from build123d import *

# Parameters (mm, degrees)
ESTRUSIONE_SOTTILE1_DEPTH    = 10
TAGLIO_ESTRUSIONE2_DEPTH     = 10
SCHIZZO3_R                   = 12.75
SCHIZZO3_R_2                 = 3.161562041
ESTRUSIONE_ESTRUSIONE1_DEPTH = 10


with BuildPart() as part:
    # Schizzo1 → Estrusione-Sottile1 (new body)
    with BuildSketch(Plane.XY):
        with BuildLine():
            Line((22.150088511, 48.999474912), (22.150088511, -48.999474912))
            ThreePointArc((22.150088511, -48.999474912), (0, -71.149563424), (-22.150088511, -48.999474912))
            Line((-22.150088511, -48.999474912), (-22.150088511, 48.999474912))
            ThreePointArc((-22.150088511, 48.999474912), (0, 71.149563424), (22.150088511, 48.999474912))
        make_face()
        with BuildLine():
            Line((12.150088511, 48.999474912), (12.150088511, -48.999474912))
            ThreePointArc((12.150088511, -48.999474912), (0, -61.149563424), (-12.150088511, -48.999474912))
            Line((-12.150088511, -48.999474912), (-12.150088511, 48.999474912))
            ThreePointArc((-12.150088511, 48.999474912), (0, 61.149563424), (12.150088511, 48.999474912))
        make_face(mode=Mode.SUBTRACT)
    extrude(amount=ESTRUSIONE_SOTTILE1_DEPTH)

    # Schizzo2 → Taglio-Estrusione2 (cut)
    with BuildSketch(Plane.XY.offset(10)):
        Polygon((-22.150088511, -48.999474912), (-17.530912976, -62.538068313), (-24.875817955, -62.538068313), (-24.875817955, -48.999474912), align=None)
    extrude(amount=-TAGLIO_ESTRUSIONE2_DEPTH, mode=Mode.SUBTRACT)

    # Schizzo3 → Estrusione-Estrusione1 (add)
    with BuildSketch(Plane.XY.offset(10)):
        with Locations((-0.05861952, -74.447142179)):
            Circle(SCHIZZO3_R)
        with Locations((-0.05861952, -74.447142179)):
            Circle(SCHIZZO3_R_2, mode=Mode.SUBTRACT)
    extrude(amount=-ESTRUSIONE_ESTRUSIONE1_DEPTH)


solid = part.part
Work out the finished part from the listing and answer in its coordinate system (mm). A direction names the side the tool comes from. Round coordinates to 2 decimals unless told otherwise and drop trailing zeros. Order: outer loops, then holes, each group sorted by start corner. A loop starts at its lowest first (then second) coordinate and runs counter-clockwise, first axis right, second up. Notation, with made-up numbers: M 1.5,2.5 L 44.5,2.5 A19 ccw 44.5,13.5 Z; hole C 59.25,-36 d5. An arc over 180 degrees is marked long. Put each result on its own line as item: value. Start each with the question number.
Q1. Section C-C, the plane z = 2 is taken. Write down the section's boundary in (x, y), and give its area (3 significant figures).
Q2. Flat-ended cylindrical pins translate along their axes: pin 1 (6 mm diameter, centred on x = 16.5, z = 1.5, fed in from +Y); pin 2 (6 mm diameter, centred on x = 5, z = 7, fed in from +Y); pin 3 (1.5 mm diameter, centred on x = -16.5, z = 6.5, fed in from +Y); pin 4 (5.5 mm diameter, centred on x = -0.06, y = -74.45, fed in from +Z). Find the tip coordinate at first contact, or state that the pin passes through.
Q3. For a pull along Y with two mould halves and no side action, classify faces 4 (the cylindrical face through (-0.47, -71.312, 5.07)), 5 (the cylindrical face through (-0.487, 71.144, 4.93)), 6 (the flat face through (14, -7, 0)) as pulls with the +Y half, pulls with the -Y half, needs draft (parallel to the pull), parting line crosses it, or undercut.
Q4. Section D-D, the plane x = 7 is taken. Write down the section's boundary in (y, z).
Q5. Straight lines are drawn through the part: L1, parallel to X at y = -37, z = 0.5; L2, parallel to Y at x = 0.5, z = 6; L3, parallel to Y at x = -1.5, z = 8. For each, find the intervals that lie inside material, in ascending order. Write a range as [from, to].
Q6. A tool of negligible diameter and unlimited length cuts with its end or side. For faces 1 (the flat face through (-12.15, -1, 5)), 2 (the flat face through (-22.15, -1, 5)), 3 (the cylindrical face through (-14.56, -65.69, 4.93)), from which of +Z, -Z, +X, -X, +Y, -Y can it reach the whole face along a straight path? Write none if from no direction.
Q7. Section B-B, the plane x = 0 is taken. Write down the section's boundary in (y, z), and give its area (3 significant figures).
Q8. Section A-A, the plane y = 45 is taken. Write down the section's boundary in (x, z), and give its area (3 significant figures).
Findings below:
1. outline: M -22.15,-49 L -17.53,-62.54 A22.15 ccw -11.14,-68.14 A12.75 ccw long 11.05,-68.19 A22.15 ccw 22.15,-49 L 22.15,49 A22.15 ccw -22.15,49 Z; hole M -12.15,-49 A12.15 ccw 12.15,-49 L 12.15,49 A12.15 ccw -12.15,49 Z; hole C -0.06,-74.45 d6.32
1. area: 3,360 mm^2
2. pin 1: stops at y = 66.56
2. pin 2: stops at y = 71.06
2. pin 3: stops at y = 64.57
2. pin 4: passes through
3. face 4: undercut
3. face 5: pulls with the +Y half
3. face 6: needs draft
4. outline: M -85.06,0 L -58.93,0 L -58.93,10 L -85.06,10 Z; M 58.93,0 L 70.01,0 L 70.01,10 L 58.93,10 Z
5. L1: x = [-22.15, -12.15], [12.15, 22.15]
5. L2: y = [-87.18, -77.56], [-71.34, -61.14], [61.14, 71.14]
5. L3: y = [-87.12, -77.26], [-71.63, -61.06], [61.06, 71.1]
6. face 1: +Z, -Z
6. face 2: +Z, -Z, -X, +Y, -Y
6. face 3: +Z, -Z, -X
7. outline: M -87.2,0 L -77.61,0 L -77.61,10 L -87.2,10 Z; M -71.29,0 L -61.15,0 L -61.15,10 L -71.29,10 Z; M 61.15,0 L 71.15,0 L 71.15,10 L 61.15,10 Z
7. area: 297 mm^2
8. outline: M -22.15,0 L -12.15,0 L -12.15,10 L -22.15,10 Z; M 12.15,0 L 22.15,0 L 22.15,10 L 12.15,10 Z
8. area: 200 mm^2
